For this review, use the dimensioned drawing (mm, ordinates from the lowest corner) and the shaded views. Round coordinates to 2 decimals unless told otherwise and drop trailing zeros. Write each loop counter-clockwise with the first axis right and the second up, starting at its lowest first coordinate (ties: lowest second). Pieces come first, ordered by that corner, then holes. Notation, with made-up numbers: M 6,1.5 L 12,1.5 A12 cw 12,19.5 Z; hole C 65.25,34.5 d3. An arc over 180 degrees is marked long. Use CSV: the item, a comma, the result in double quotes.
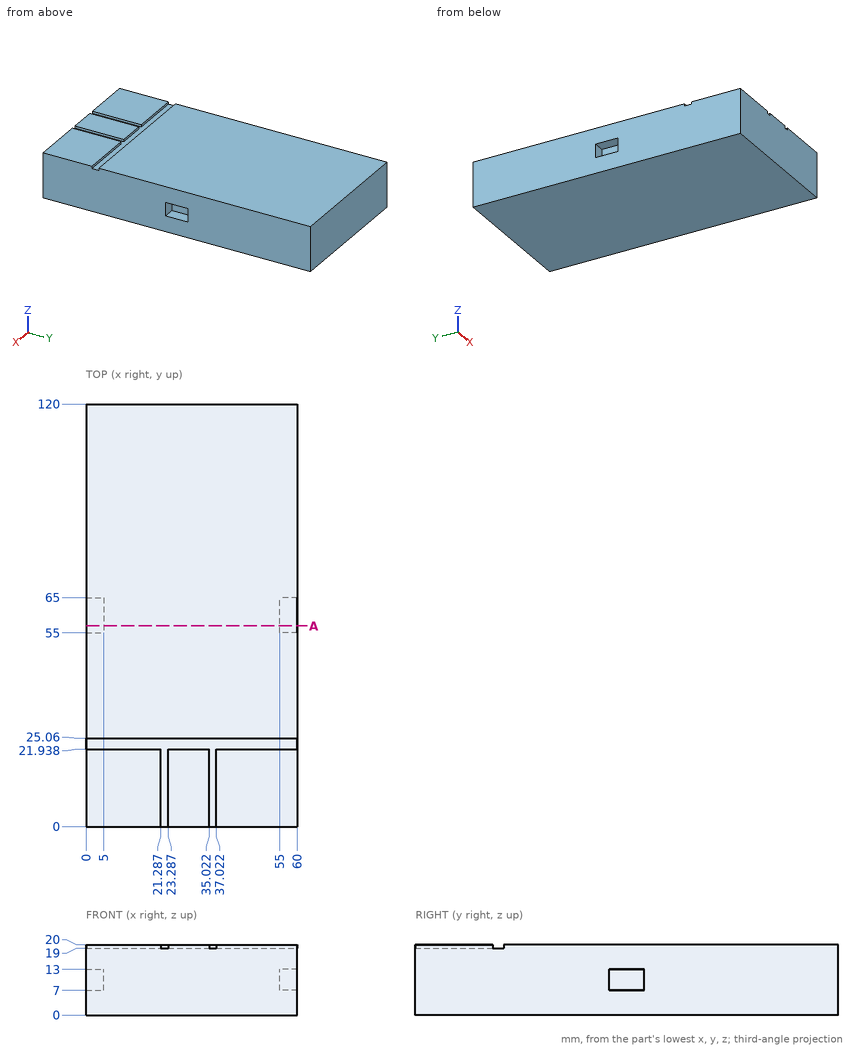
1) For pin 1 Ø4 at (x, y) = (58, 59) entering from -Z, flat-tipped, find the tip position at first contact; note if it passes through.
Answers:
pin 1,"z = 0"
2) Wall thickness on line 1 along Y through (x, z) = (56, 12.5); line 2 along X through (y, z) = (64.5, 10.25): over which ranges is each line inside the solid? List them lowest first. Write a range as [from, to].
Answers:
line 1,"[0, 55], [65, 120]"
line 2,"[5, 55]"
3) Add section A-A on y = 57. Write out the cut boundary in (x, z), then the cut area to 3 significant figures.
Answers:
outline,"M 0,0 L 60,0 L 60,7 L 55,7 L 55,13 L 60,13 L 60,20 L 0,20 L 0,13 L 5,13 L 5,7 L 0,7 Z"
area,"1,140 mm²"
